Here's the drawing with two shaded views (mm, measured from the low corner). I have some questions. A direction names the side the tool comes from. Round coordinates to 2 decimals unless told otherwise and drop trailing zeros. Order: outer loops, then holes, each group sorted by start corner. A loop starts at its lowest first (then second) coordinate and runs counter-clockwise, first axis right, second up.
Q1. Will these pins go through, and if not, where does the flat tip stop? P1, Ø4, axis at x = 10, z = 2.5, coming from the -Y side; P2, Ø4.5, axis at y = 20, z = 25.5, coming from the -X side; P3, Ø5, axis at x = 7.5, y = 14, coming from the +Z side.
Q2. If we section it at A-A (y = 17.5): Please give me the cut outline in (x, z).
Q3. If we section it at B-B (z = 3.5): Please give me the cut outline in (x, y), plus the area to 3 significant figures.
Q4. If we section it at D-D (z = 18.25): Please give me the cut outline in (x, y), plus the area to 3 significant figures.
Q5. For the marked faces 1, 2 and 3, which set-ups out of +Z, -Z, +X, -X, +Y, -Y let a thin tool reach every point of the face, with its end or its side?
Q6. If I drill on line 1 (X direction, y = 1.75, z = 2.25); line 2 (Y direction, x = 52, z = 3.25); line 3 (Z direction, x = 8.5, y = 11.5), over which ranges is the centre line in solid material (lowest first)?
Q7. If we section it at C-C (x = 10): Please give me the cut outline in (y, z).
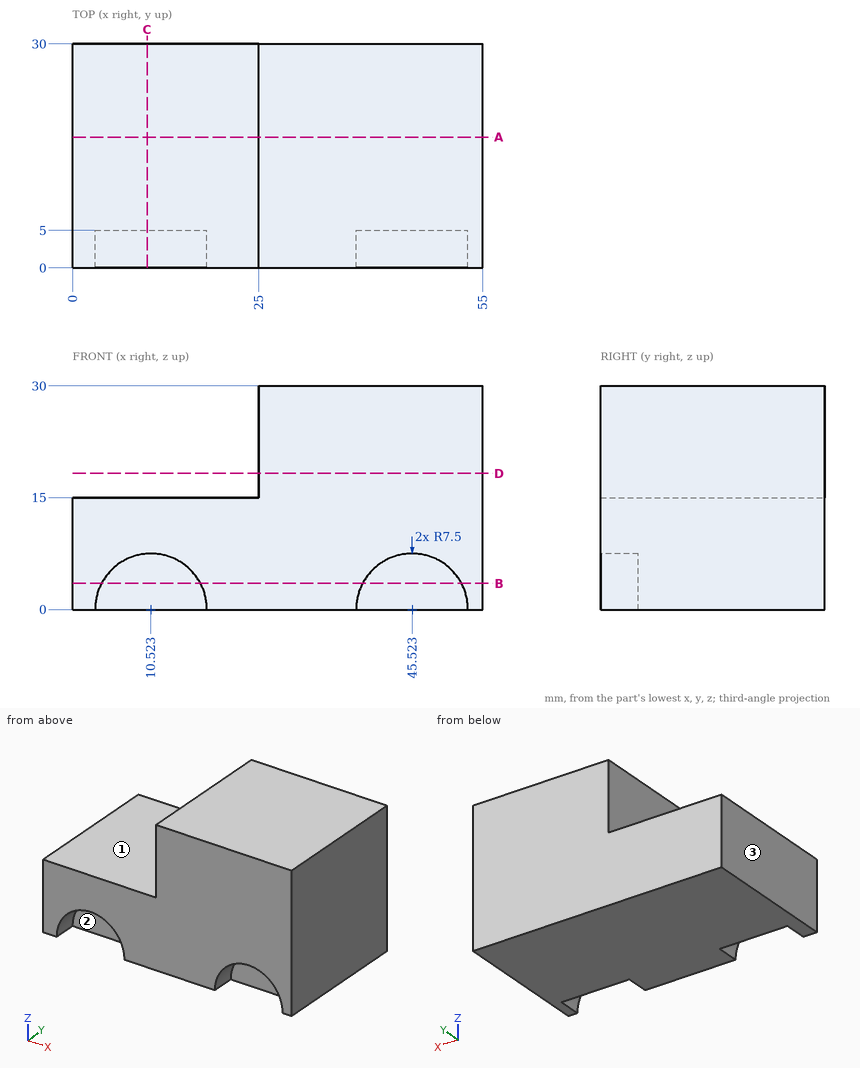
Solution:
1. P1: stops at y = 5
1. P2: stops at x = 25
1. P3: stops at z = 15
2. outline: (0, 0) - (55, 0) - (55, 30) - (25, 30) - (25, 15) - (0, 15) - close
3. outline: (0, 0) - (3.89, 0) - (3.89, 5) - (17.16, 5) - (17.16, 0) - (38.89, 0) - (38.89, 5) - (52.16, 5) - (52.16, 0) - (55, 0) - (55, 30) - (0, 30) - close
3. area: 1,520 mm2
4. outline: (25, 0) - (55, 0) - (55, 30) - (25, 30) - close
4. area: 900 mm2
5. face 1: +Z, -X, +Y, -Y
5. face 2: -Z, -Y
5. face 3: +Z, -Z, -X, +Y, -Y
6. line 1: x = 0 to 3.37, 17.68 to 38.37, 52.68 to 55
6. line 2: y = 5 to 30
6. line 3: z = 0 to 15
7. outline: (0, 7.48) - (5, 7.48) - (5, 0) - (30, 0) - (30, 15) - (0, 15) - close
